Check sheet for the modelled part. Datum: model origin and axes. Units: mm. Round coordinates to 2 decimals unless told otherwise and drop trailing zeros. Write each loop counter-clockwise with the first axis right and the second up, starting at its lowest first coordinate (ties: lowest second). Pieces come first, ordered by that corner, then holes. Notation, with made-up numbers: M -3.75,41.25 L 36.25,41.25 A13 ccw 36.25,47.25 Z; hole C -39,-18 d3. An arc over 180 degrees is marked long. Answer in a Markdown table with one row per item.
```python
from build123d import *

# Parameters (mm, degrees)
BOSS_EXTRUDE1_DEPTH = 12


with BuildPart() as part:
    # Sketch1 → Boss-Extrude1 (new body)
    with BuildSketch(Plane.XY):
        with BuildLine():
            Line((511.8067094, 188.903885219), (511.8067094, 142.299329353))
            ThreePointArc((511.8067094, 142.299329353), (511.806507744, 138.903885219), (515.20195099, 138.906348311))
            Line((515.20195099, 138.906348311), (523.8067094, 138.906348311))
            Line((523.8067094, 138.906348311), (523.8067094, 138.319810176))
            Line((523.8067094, 138.319810176), (523.8067094, 88.903885219))
            Line((523.8067094, 88.903885219), (518.8067094, 88.903885219))
            Line((518.8067094, 88.903885219), (515.20195099, 88.903885219))
            ThreePointArc((515.20195099, 88.903885219), (511.806507744, 88.906348311), (511.8067094, 85.510904177))
            Line((511.8067094, 85.510904177), (511.8067094, 42.296866261))
            ThreePointArc((511.8067094, 42.296866261), (511.806507744, 38.901422127), (515.20195099, 38.903885219))
            Line((515.20195099, 38.903885219), (518.8067094, 38.903885219))
            Line((518.8067094, 38.903885219), (523.8067094, 38.903885219))
            Line((523.8067094, 38.903885219), (523.8067094, -11.096114781))
            Line((523.8067094, -11.096114781), (518.8067094, -11.096114781))
            Line((518.8067094, -11.096114781), (515.20195099, -11.096114781))
            ThreePointArc((515.20195099, -11.096114781), (511.806507744, -11.093651689), (511.8067094, -14.489095823))
            Line((511.8067094, -14.489095823), (511.8067094, -57.703133739))
            ThreePointArc((511.8067094, -57.703133739), (511.806507744, -61.098577873), (515.20195099, -61.096114781))
            Line((515.20195099, -61.096114781), (518.8067094, -61.096114781))
            Line((518.8067094, -61.096114781), (523.8067094, -61.096114781))
            Line((523.8067094, -61.096114781), (523.8067094, -111.096114781))
            Line((523.8067094, -111.096114781), (518.8067094, -111.096114781))
            Line((518.8067094, -111.096114781), (515.20195099, -111.096114781))
            ThreePointArc((515.20195099, -111.096114781), (511.806507744, -111.093651689), (511.8067094, -114.489095823))
            Line((511.8067094, -114.489095823), (511.8067094, -161.096114781))
            Line((511.8067094, -161.096114781), (-613.922135209, -161.096114781))
            Line((-613.922135209, -161.096114781), (-613.922135209, -114.489095823))
            ThreePointArc((-613.922135209, -114.489095823), (-613.921933554, -111.093651689), (-617.3173768, -111.096114781))
            Line((-617.3173768, -111.096114781), (-620.922135209, -111.096114781))
            Line((-620.922135209, -111.096114781), (-625.922135209, -111.096114781))
            Line((-625.922135209, -111.096114781), (-625.922135209, -61.096114781))
            Line((-625.922135209, -61.096114781), (-620.922135209, -61.096114781))
            Line((-620.922135209, -61.096114781), (-617.3173768, -61.096114781))
            ThreePointArc((-617.3173768, -61.096114781), (-613.921933554, -61.098577873), (-613.922135209, -57.703133739))
            Line((-613.922135209, -57.703133739), (-613.922135209, -14.489095823))
            ThreePointArc((-613.922135209, -14.489095823), (-613.921933554, -11.093651689), (-617.3173768, -11.096114781))
            Line((-617.3173768, -11.096114781), (-620.922135209, -11.096114781))
            Line((-620.922135209, -11.096114781), (-625.922135209, -11.096114781))
            Line((-625.922135209, -11.096114781), (-625.922135209, 38.903885219))
            Line((-625.922135209, 38.903885219), (-620.922135209, 38.903885219))
            Line((-620.922135209, 38.903885219), (-617.3173768, 38.903885219))
            ThreePointArc((-617.3173768, 38.903885219), (-613.921933554, 38.901422127), (-613.922135209, 42.296866261))
            Line((-613.922135209, 42.296866261), (-613.922135209, 85.510904177))
            ThreePointArc((-613.922135209, 85.510904177), (-613.921933554, 88.906348311), (-617.3173768, 88.903885219))
            Line((-617.3173768, 88.903885219), (-620.922135209, 88.903885219))
            Line((-620.922135209, 88.903885219), (-625.922135209, 88.903885219))
            Line((-625.922135209, 88.903885219), (-625.922135209, 138.319810176))
            Line((-625.922135209, 138.319810176), (-625.922135209, 138.906348311))
            Line((-625.922135209, 138.906348311), (-617.3173768, 138.906348311))
            ThreePointArc((-617.3173768, 138.906348311), (-613.921933554, 138.903885219), (-613.922135209, 142.299329353))
            Line((-613.922135209, 142.299329353), (-613.922135209, 188.903885219))
            Line((-613.922135209, 188.903885219), (511.8067094, 188.903885219))
        make_face()
        with BuildLine():
            Line((-48.336173874, 138.906348311), (-53.779251936, 138.906348311))
            ThreePointArc((-53.779251936, 138.906348311), (-57.55476918, 139.403404586), (-57.057712905, 135.627887342))
            Line((-57.057712905, 135.627887342), (-57.057712905, 92.18480928))
            ThreePointArc((-57.057712905, 92.18480928), (-57.55476918, 88.409292036), (-53.779251936, 88.906348311))
            Line((-53.779251936, 88.906348311), (-48.336173874, 88.906348311))
            ThreePointArc((-48.336173874, 88.906348311), (-44.56065663, 88.409292036), (-45.057712905, 92.18480928))
            Line((-45.057712905, 92.18480928), (-45.057712905, 135.627887342))
            ThreePointArc((-45.057712905, 135.627887342), (-44.56065663, 139.403404586), (-48.336173874, 138.906348311))
        make_face(mode=Mode.SUBTRACT)
        with BuildLine():
            Line((-48.345370421, 38.903885219), (-53.770055388, 38.903885219))
            ThreePointArc((-53.770055388, 38.903885219), (-57.548209819, 39.423547352), (-57.057712905, 35.641496003))
            Line((-57.057712905, 35.641496003), (-57.057712905, -7.833725565))
            ThreePointArc((-57.057712905, -7.833725565), (-57.548209819, -11.615776914), (-53.770055388, -11.096114781))
            Line((-53.770055388, -11.096114781), (-48.345370421, -11.096114781))
            ThreePointArc((-48.345370421, -11.096114781), (-44.567215991, -11.615776914), (-45.057712905, -7.833725565))
            Line((-45.057712905, -7.833725565), (-45.057712905, 35.641496003))
            ThreePointArc((-45.057712905, 35.641496003), (-44.567215991, 39.423547352), (-48.345370421, 38.903885219))
        make_face(mode=Mode.SUBTRACT)
        with BuildLine():
            Line((-48.336173874, -61.096114781), (-53.779251936, -61.096114781))
            ThreePointArc((-53.779251936, -61.096114781), (-57.55476918, -60.599058506), (-57.057712905, -64.37457575))
            Line((-57.057712905, -64.37457575), (-57.057712905, -107.817653812))
            ThreePointArc((-57.057712905, -107.817653812), (-57.55476918, -111.593171056), (-53.779251936, -111.096114781))
            Line((-53.779251936, -111.096114781), (-48.336173874, -111.096114781))
            ThreePointArc((-48.336173874, -111.096114781), (-44.56065663, -111.593171056), (-45.057712905, -107.817653812))
            Line((-45.057712905, -107.817653812), (-45.057712905, -64.37457575))
            ThreePointArc((-45.057712905, -64.37457575), (-44.56065663, -60.599058506), (-48.336173874, -61.096114781))
        make_face(mode=Mode.SUBTRACT)
    extrude(amount=BOSS_EXTRUDE1_DEPTH)


solid = part.part
```
1. Go/stop test with flat-tipped pins: pin 1 (7 mm diameter, centred on x = -619.5, z = 9, fed in from -Y); pin 2 (2.5 mm diameter, centred on x = -623, z = 5, fed in from +Y); pin 3 (6 mm diameter, centred on y = -28.5, z = 4.5, fed in from +X). Record where each tip stops, or that it passes through.
Found:
| item | result |
|---|---|
| pin 1 | stops at y = -111.1 |
| pin 2 | stops at y = 138.91 |
| pin 3 | stops at x = 511.81 |
2. Section check B-B, the plane y = 168.5. Record the cut outline in (x, z), and give its area (3 significant figures).
Found:
| item | result |
|---|---|
| outline | M -613.92,0 L 511.81,0 L 511.81,12 L -613.92,12 Z |
| area | 13,500 mm2 |
3. Scan lines: L1, parallel to X at y = -5, z = 3; L2, parallel to X at y = 38.5, z = 3.5; L3, parallel to X at y = -10, z = 4.75. Record each from-to range of solid material in increasing order.
Found:
| item | result |
|---|---|
| L1 | x = -625.92 to -57.06, -45.06 to 523.81 |
| L2 | x = -625.92 to -616.78, -614.45 to -58.13, -43.99 to 512.34, 514.67 to 523.81 |
| L3 | x = -625.92 to -58.26, -43.86 to 523.81 |
4. Section check A-A, the plane z = 4. Count the separate pieces of the cut face and the enclosed holes in it, and give its area (3 significant figures).
Found:
| item | result |
|---|---|
| separate pieces | 1 |
| enclosed holes | 3 |
| area | 396,000 mm2 |
